Input: part model. Units: mm. Frame: model coordinates. A direction names the side the tool comes from. Give positions to 0.01 mm unless a question says otherwise; leave off trailing zeros. Write each loop counter-clockwise with the first axis right and the second up, starting at its lowest first coordinate (ties: lowest second). Pieces come first, ordered by that corner, then holes. Notation, with made-up numbers: (-29, 67.5) - (13, 67.5) arc R20 cw to (13, 99.5) - close; hole circle Ø10 at (85.5, -29). An arc over 180 degrees is marked (long way). Use a Markdown table: item, result. Add a question column.
1. Mould query, pull axis Y, two halves, no side actions, for faces 5 (the cylindrical face through (-26.479, 52.234, -14.239)), 6 (the cylindrical face through (26.521, 52.234, -14.239)), 7 (the flat face through (0, 46, 2.409)), 8 (the flat face through (-24, 49, -12)). Classes: released by +Y, released by -Y, zero draft, split by the parting line, or undercut.
2. Section query A-A, the plane x = 1. Return loops of the section in (y, z), plus the area to 3 significant figures.
3. Pin query (flat end, axial travel): pin 1 (6 mm diameter, centred on y = 62.5, z = -7.5, fed in from +X); pin 2 (1.5 mm diameter, centred on x = 2, z = 0.5, fed in from +Y); pin 3 (5 mm diameter, centred on x = -6.5, y = 19, fed in from -Z). Return the tip coordinate at first contact, or that it passes through.
4. Section query C-C, the plane z = -2.5. Return loops of the section in (x, y).
5. Material intervals for probe 1 along X at (y, z) = (58.5, -2); probe 2 along X at (y, z) = (14, -9.5); probe 3 along Y at (x, z) = (9, -3), sorted ascending.
6. Section query D-D, the plane z = -12. Count the separate pieces of the cut face and the enclosed holes in it, plus the area to 3 significant figures.
7. Section query B-B, the plane y = 53. Return loops of the section in (x, z).
8. Set-up query: faces 1 (the flat face through (-10.3, 49, -3.5)), 2 (the flat face through (2, 47, -14)), 3 (the flat face through (0, 10, 7.609)), 4 (the flat face through (-8, 75.5, 4)). Return all of +Z, -Z, +X, -X, +Y, -Y with unobstructed straight access to the full face (end or side cutting, diameter ignored); none if empty.
```python
from build123d import *

# Parameters (mm, degrees)
SALIENTE_EXTRUIR1_DEPTH   = 45
SALIENTE_EXTRUIR1_2_DEPTH = 45
SALIENTE_EXTRUIR2_DEPTH   = 3
SALIENTE_EXTRUIR3_START   = -45
SALIENTE_EXTRUIR3_DEPTH   = 2
CROQUIS4_W                = 3
CROQUIS4_H                = 10
SALIENTE_EXTRUIR4_DEPTH   = 10
CROQUIS5_R                = 2
CORTAR_EXTRUIR1_DEPTH     = 87.967390625
CHAFL_N1_SIZE             = 3
CORTAR_EXTRUIR3_DEPTH     = 77.377856949
SALIENTE_EXTRUIR7_DEPTH   = 54
CROQUIS6_W                = 15
CROQUIS6_H                = 20
CORTAR_EXTRUIR5_DEPTH     = 74.806009458
CORTAR_EXTRUIR6_DEPTH     = 74.806009458
CORTAR_EXTRUIR7_DEPTH     = 77.377856949
CROQUIS16_W               = 12.6
CROQUIS16_H               = 3
CORTAR_EXTRUIR8_DEPTH     = 5
CROQUIS18_W               = 3
CROQUIS18_H               = 20
SALIENTE_EXTRUIR8_DEPTH   = 27.5
CORTAR_EXTRUIR9_REACH     = 90.622
CROQUIS21_W               = 4
CROQUIS21_H               = 10
CORTAR_EXTRUIR10_DEPTH    = 3
CROQUIS22_R               = 1.6
CORTAR_EXTRUIR11_DEPTH    = 89.621555367
CHAFL_N2_SIZE             = 2


with BuildPart() as part:
    # Croquis1 → Saliente-Extruir1 (new body)
    with BuildSketch(Plane(origin=(0, 0, 0), x_dir=(1, 0, 0), z_dir=(0, 1, 0))):
        Polygon((-26, 17.391304348), (-26, 8.344494697), (-7.5, -6.655505303), (-7.5, -32.608695652), (-9.5, -32.608695652), (-9.5, -7.608695652), (-28, 7.391304348), (-28, 17.391304348), align=None)
    extrude(amount=SALIENTE_EXTRUIR1_DEPTH)



with BuildPart() as body_2:
    # Croquis1 → Saliente-Extruir1 2 (new body)
    with BuildSketch(Plane(origin=(0, 0, 0), x_dir=(1, 0, 0), z_dir=(0, 1, 0))):
        Polygon((7.5, -6.655505303), (7.5, -32.608695652), (9.5, -32.608695652), (9.5, -7.608695652), (28, 7.391304348), (28, 17.391304348), (26, 17.391304348), (26, 8.344494697), align=None)
    extrude(amount=SALIENTE_EXTRUIR1_2_DEPTH)


with BuildPart() as part_1:
    add(part.part)

    add(body_2.part)  # Saliente-Extruir2 merges body 2
    # Croquis2 → Saliente-Extruir2 (add)
    with BuildSketch(Plane(origin=(0, 45, 0), x_dir=(1, 0, 0), z_dir=(0, 1, 0))):
        Polygon((-9.5, -32.608695652), (9.5, -32.608695652), (9.5, -7.608695652), (28, 7.391304348), (28, 17.391304348), (-28, 17.391304348), (-28, 7.391304348), (-9.5, -7.608695652), align=None)
    extrude(amount=SALIENTE_EXTRUIR2_DEPTH)

    # Croquis2<2> → Saliente-Extruir3 (add)
    with BuildSketch(Plane(origin=(0, 45, 0), x_dir=(1, 0, 0), z_dir=(0, 1, 0)).offset(SALIENTE_EXTRUIR3_START)):
        Polygon((-9.5, -32.608695652), (9.5, -32.608695652), (9.5, -7.608695652), (28, 7.391304348), (28, 17.391304348), (-28, 17.391304348), (-28, 7.391304348), (-9.5, -7.608695652), align=None)
    extrude(amount=-SALIENTE_EXTRUIR3_DEPTH)

    # Croquis4 → Saliente-Extruir4 (add)
    with BuildSketch(Plane(origin=(0, 48, 0), x_dir=(1, 0, 0), z_dir=(0, 1, 0))):
        with Locations((-26.5, 12.391304348)):
            Rectangle(CROQUIS4_W, CROQUIS4_H)
        with Locations((26.5, 12.391304348)):
            Rectangle(CROQUIS4_W, CROQUIS4_H)
    extrude(amount=SALIENTE_EXTRUIR4_DEPTH)

    # Croquis5 → Cortar-Extruir1 (cut, through all)
    with BuildSketch(Plane(origin=(28, 0, 0), x_dir=(0, 0, -1), z_dir=(1, 0, 0))):
        with Locations((12.391304348, 53)):
            Circle(CROQUIS5_R)
    extrude(amount=-CORTAR_EXTRUIR1_DEPTH, mode=Mode.SUBTRACT)

    # Chaflán1
    chafl_n1_edges = [part_1.edges().sort_by_distance(p)[0] for p in [
        (-26.5, 58, -7.391304348),
        (-26.5, 58, -17.391304348),
        (26.5, 58, -17.391304348),
        (26.5, 58, -7.391304348),
    ]]
    chamfer(chafl_n1_edges, length=CHAFL_N1_SIZE)

    # Croquis7 → Cortar-Extruir3 (cut, through all)
    with BuildSketch(Plane(origin=(9.5, 0, 0), x_dir=(0, 0, -1), z_dir=(1, 0, 0))):
        Polygon((-32.608695652, -2), (-11.608695652, 48), (-32.608695652, 48), align=None)
    extrude(amount=-CORTAR_EXTRUIR3_DEPTH, mode=Mode.SUBTRACT)

    # Croquis13 → Saliente-Extruir7 (add)
    with BuildSketch(Plane(origin=(-26, 0, 0), x_dir=(0, 0, -1), z_dir=(1, 0, 0))):
        Polygon((17.391304348, 45), (-12.868695652, 45), (-14.968695652, 40), align=None)
        Polygon((17.391304348, 0), (-31.768695652, 0), (-18.748695652, 31), align=None)
    extrude(amount=SALIENTE_EXTRUIR7_DEPTH)

    # Croquis6 → Cortar-Extruir5 (cut, through all)
    with BuildSketch(Plane.XZ.offset(2)):
        with Locations((0, 17.608695652)):
            Rectangle(CROQUIS6_W, CROQUIS6_H)
    extrude(amount=-CORTAR_EXTRUIR5_DEPTH, mode=Mode.SUBTRACT)

    # Croquis14 → Cortar-Extruir6 (cut, through all)
    with BuildSketch(Plane.XZ.offset(2)):
        Polygon((-28, -7.391304348), (-9.5, 7.608695652), (-9.5, 32.608695652), (-28, 32.608695652), align=None)
        Polygon((28, -7.391304348), (9.5, 7.608695652), (9.5, 32.608695652), (28, 32.608695652), align=None)
    extrude(amount=-CORTAR_EXTRUIR6_DEPTH, mode=Mode.SUBTRACT)

    # Croquis15 → Cortar-Extruir7 (cut, through all)
    with BuildSketch(Plane(origin=(9.5, 0, 0), x_dir=(0, 0, -1), z_dir=(1, 0, 0))):
        Polygon((-27.608695652, -2), (-27.608695652, 9.904761905), (-32.608695652, -2), align=None)
    extrude(amount=-CORTAR_EXTRUIR7_DEPTH, mode=Mode.SUBTRACT)

    # Croquis16 → Cortar-Extruir8 (cut)
    with BuildSketch(Plane(origin=(0, 48, 0), x_dir=(1, 0, 0), z_dir=(0, 1, 0))):
        with Locations((0, -0.908695652)):
            Rectangle(CROQUIS16_W, CROQUIS16_H)
    extrude(amount=-CORTAR_EXTRUIR8_DEPTH, mode=Mode.SUBTRACT)

    # Croquis18 → Saliente-Extruir8 (add)
    with BuildSketch(Plane(origin=(0, 48, 0), x_dir=(1, 0, 0), z_dir=(0, 1, 0))):
        with Locations((-7.8, 3.591304348)):
            Rectangle(CROQUIS18_W, CROQUIS18_H)
        with Locations((7.8, 3.591304348)):
            Rectangle(CROQUIS18_W, CROQUIS18_H)
    extrude(amount=SALIENTE_EXTRUIR8_DEPTH)

    # Cortar-Extruir9: up to this face of the body (flat: up to its plane)
    cortar_extruir9_end = Plane(part_1.part.faces().sort_by_distance((9.3, 61.75, -3.591304348))[0])
    # Croquis20 → Cortar-Extruir9 (cut, up to the picked face)
    with BuildSketch(Plane.ZY.offset(9.3), mode=Mode.PRIVATE) as cortar_extruir9_sk1:
        Polygon((2.408695652, 75.5), (-13.591304348, 52), (-13.591304348, 75.5), align=None)
    cortar_extruir9_tool1 = split(extrude(cortar_extruir9_sk1.sketch, amount=-CORTAR_EXTRUIR9_REACH, mode=Mode.PRIVATE), bisect_by=cortar_extruir9_end, keep=Keep.BOTH, mode=Mode.PRIVATE)
    add(cortar_extruir9_tool1.solids().sort_by(Axis((-9.3, 67.666667, -8.257971), (1, 0, 0)))[0], mode=Mode.SUBTRACT)

    # Croquis21 → Cortar-Extruir10 (cut)
    with BuildSketch(Plane(origin=(0, 48, 0), x_dir=(1, 0, 0), z_dir=(0, 1, 0))):
        with Locations((0, 14.771116856)):
            Rectangle(CROQUIS21_W, CROQUIS21_H)
    extrude(amount=-CORTAR_EXTRUIR10_DEPTH, mode=Mode.SUBTRACT)

    # Croquis22 → Cortar-Extruir11 (cut, through all)
    with BuildSketch(Plane(origin=(9.3, 0, 0), x_dir=(0, 0, -1), z_dir=(1, 0, 0))):
        with Locations((-3.908695652, 72.518591358)):
            Circle(CROQUIS22_R)
    extrude(amount=-CORTAR_EXTRUIR11_DEPTH, mode=Mode.SUBTRACT)

    # Chaflán2
    # the kernel refuses this chamfer: 2 mm, written as the material it adds along each edge
    with BuildSketch(Plane(origin=(-25, 48, -17.391304348), x_dir=(0.9996219169112968, -0.027495876610585647, 0), z_dir=(0, 0, 1)), Plane(origin=(25, 48, -17.391304348), x_dir=(0.027495876610585647, 0.9996219169112968, 0), z_dir=(0, 0, 1))) as chafl_n2_piece_1:
        Polygon((CHAFL_N2_SIZE * 0.999621916911, CHAFL_N2_SIZE * 0.0274958766106), (-CHAFL_N2_SIZE * 0.0274958766106, CHAFL_N2_SIZE * 0.999621916911), (0, 0), align=None)
    extrude(amount=10)
    with BuildSketch(Plane(origin=(-9.3, 48, 6.408695652), x_dir=(-0.9996219169112968, -0.027495876610585623, 0), z_dir=(0, 0, -1))) as chafl_n2_piece_2_section:
        Polygon((CHAFL_N2_SIZE * 0.999621916911, CHAFL_N2_SIZE * 0.0274958766106), (-CHAFL_N2_SIZE * 0.0274958766106, CHAFL_N2_SIZE * 0.999621916911), (0, 0), align=None)
    chafl_n2_piece_2 = extrude(amount=20, mode=Mode.PRIVATE)
    chafl_n2_piece_2 = split(chafl_n2_piece_2, bisect_by=Plane(origin=(-15.34165394, 48.600071078, 2.872219484), z_dir=(0.6298019584212193, 0, -0.7767557487195037)), keep=Keep.TOP, mode=Mode.PRIVATE)
    add(chafl_n2_piece_2)
    with BuildSketch(Plane(origin=(9.3, 48, 6.408695652), x_dir=(0.9996219169112968, -0.027495876610585623, 0), z_dir=(0, 0, -1))) as chafl_n2_piece_3_section:
        Polygon((CHAFL_N2_SIZE * 0.999621916911, -CHAFL_N2_SIZE * 0.0274958766106), (-CHAFL_N2_SIZE * 0.0274958766106, -CHAFL_N2_SIZE * 0.999621916911), (0, 0), align=None)
    chafl_n2_piece_3 = extrude(amount=20, mode=Mode.PRIVATE)
    chafl_n2_piece_3 = split(chafl_n2_piece_3, bisect_by=Plane(origin=(15.34165394, 48.600071078, 2.872219484), z_dir=(-0.6298019584212193, 0, -0.7767557487195037)), keep=Keep.TOP, mode=Mode.PRIVATE)
    add(chafl_n2_piece_3)


solid = part_1.part
```
Result sheet:
| question | item | result |
|---|---|---|
| 1 | face 5 | undercut |
| 1 | face 6 | undercut |
| 1 | face 7 | zero draft |
| 1 | face 8 | released by +Y |
| 2 | outline | (-2, -17.39) - (0, -17.39) - (21.44, 7.61) - (-2, 7.61) - close; (41.14, 7.61) - (45, -17.39) - (45, -9.77) - (48, -9.77) - (48, -0.59) - (43, -0.59) - (43, 2.41) - (48, 2.41) - (48, 7.61) - close |
| 2 | area | 403 mm² |
| 3 | pin 1 | stops at x = 9.3 |
| 3 | pin 2 | stops at y = 43 |
| 3 | pin 3 | stops at z = 1.84 |
| 4 | outline | (-21.97, -2) - (21.97, -2) - (21.97, 48) - (11.3, 48) - (9.3, 50) - (9.3, 68.29) - (6.3, 68.29) - (6.3, 48) - (-6.3, 48) - (-6.3, 68.29) - (-9.3, 68.29) - (-9.3, 50) - (-11.3, 48) - (-21.97, 48) - close; hole (-18.79, 12.77) - (18.79, 12.77) - (18.79, 42.7) - (-18.79, 42.7) - close |
| 5 | probe 1 | x = -9.3 to -6.3, 6.3 to 9.3 |
| 5 | probe 2 | x = -28 to -26, 26 to 28 |
| 5 | probe 3 | y = -2 to 12.34, 42.78 to 67.56 |
| 6 | separate pieces | 3 |
| 6 | enclosed holes | 1 |
| 6 | area | 814 mm² |
| 7 | outline | (-28, -17.39) - (-25, -17.39) - (-25, -14.39) - (-28, -14.39) - close; (-28, -10.39) - (-25, -10.39) - (-25, -7.39) - (-28, -7.39) - close; (-9.3, -12.91) - (-6.3, -12.91) - (-6.3, 6.41) - (-9.3, 6.41) - close; (6.3, -12.91) - (9.3, -12.91) - (9.3, 6.41) - (6.3, 6.41) - close; (25, -17.39) - (28, -17.39) - (28, -14.39) - (25, -14.39) - close; (25, -10.39) - (28, -10.39) - (28, -7.39) - (25, -7.39) - close |
| 8 | face 1 | +Z, -Z, +Y |
| 8 | face 2 | -Z, +Y |
| 8 | face 3 | +Z, +Y, -Y |
| 8 | face 4 | +Z, -Z, +X, -X, +Y |
